Study the drawing (mm; zero at the part's minimum x, y, z) and answer. Give positions to 0.01 mm unless a question says otherwise; leave off trailing zeros. Order: outer loops, then holes, each group sorted by start corner. A loop starts at its lowest first (then second) coordinate and runs counter-clockwise, first axis right, second up. Notation, with made-up numbers: (-35.5, 2) - (-14.5, 2) arc R16 ccw to (-14.5, 26) - close; hole circle Ø7 at (-2.75, -16). An arc over 180 degrees is marked (long way). Use CSV: the item, a comma, the result in double quotes.
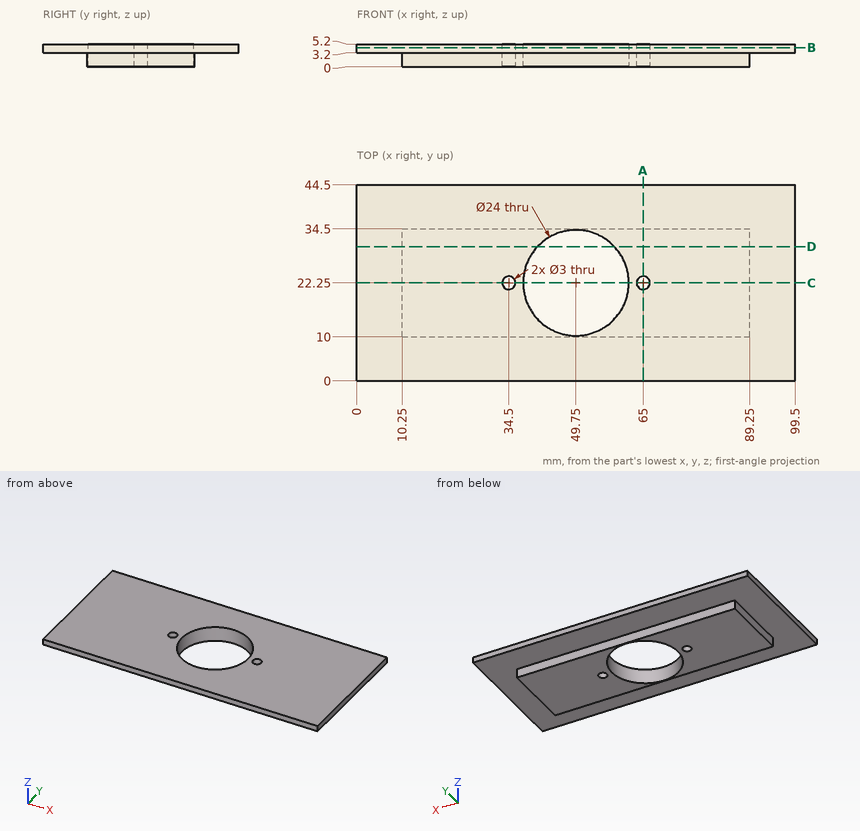
Item 1: Each of these flat-tipped pins is pushed along its axis until it touches: pin 1 (21.5 mm diameter, centred on x = 49.75, y = 22.25, fed in from -Z); pin 2 (3 mm diameter, centred on x = 54.5, z = 1.5, fed in from +Y); pin 3 (1 mm diameter, centred on y = 25, z = 1, fed in from +X); pin 4 (2 mm diameter, centred on x = 16.5, y = 39, fed in from -Z). Where does it stop, or does it pass through?
Taken from the geometry:
pin 1,"through"
pin 2,"y = 34.5"
pin 3,"x = 89.25"
pin 4,"z = 3.2"
Item 2: Find the intervals of material crossed by line 1 along Y through (x, z) = (49.75, 2.9); line 2 along Y through (x, z) = (34.5, 3.3); line 3 along Z through (x, y) = (76, 6.5), in increasing order.
Taken from the geometry:
line 1,"10 to 10.25, 34.25 to 34.5"
line 2,"0 to 20.75, 23.75 to 44.5"
line 3,"3.2 to 5.2"
Item 3: The part is cut by section D-D (y = 30.5). Give the vertices of the cut face in (x, z).
Taken from the geometry:
outline,"(0, 3.2) - (10.25, 3.2) - (10.25, 0) - (41.04, 0) - (41.04, 5.2) - (0, 5.2) - close; (58.46, 0) - (89.25, 0) - (89.25, 3.2) - (99.5, 3.2) - (99.5, 5.2) - (58.46, 5.2) - close"
Item 4: The part is cut by section A-A (x = 65). Give the vertices of the cut face in (y, z).
Taken from the geometry:
outline,"(0, 3.2) - (10, 3.2) - (10, 0) - (20.75, 0) - (20.75, 5.2) - (0, 5.2) - close; (23.75, 0) - (34.5, 0) - (34.5, 3.2) - (44.5, 3.2) - (44.5, 5.2) - (23.75, 5.2) - close"
Item 5: The part is cut by section C-C (y = 22.25). Give the vertices of the cut face in (x, z).
Taken from the geometry:
outline,"(0, 3.2) - (10.25, 3.2) - (10.25, 0) - (33, 0) - (33, 5.2) - (0, 5.2) - close; (36, 0) - (37.75, 0) - (37.75, 5.2) - (36, 5.2) - close; (61.75, 0) - (63.5, 0) - (63.5, 5.2) - (61.75, 5.2) - close; (66.5, 0) - (89.25, 0) - (89.25, 3.2) - (99.5, 3.2) - (99.5, 5.2) - (66.5, 5.2) - close"
Item 6: The part is cut by section B-B (z = 4.4). Give the vertices of the cut face in (x, y).
Taken from the geometry:
outline,"(0, 0) - (99.5, 0) - (99.5, 44.5) - (0, 44.5) - close; hole circle Ø3 at (34.5, 22.25); hole circle Ø24 at (49.75, 22.25); hole circle Ø3 at (65, 22.25)"
